CAD build for the part. Positions are in the model's coordinates, mm. Face numbers are marked on the shaded views. A direction names the side the tool comes from. Round coordinates to 2 decimals unless told otherwise and drop trailing zeros. Loops run counter-clockwise (first coordinate to the right, second up) from the corner with the lowest first, then second, coordinate; pieces in that order, holes last.
```python
from build123d import *

# Parameters (mm, degrees)
SKETCH1_R                    = 27.5
BOSS_EXTRUDE1_DEPTH          = 50
SKETCH2_R                    = 67.5
SKETCH2_R_2                  = 14
BOSS_EXTRUDE2_DEPTH          = 28
SKETCH3_R                    = 9
CUT_EXTRUDE1_DEPTH           = 12
CUT_EXTRUDE1_DRAFT           = -7.5
CUT_EXTRUDE1_PROFILE_2_DEPTH = 12
CUT_EXTRUDE1_PROFILE_2_DRAFT = -7.5
CUT_EXTRUDE1_PROFILE_3_DEPTH = 12
CUT_EXTRUDE1_PROFILE_3_DRAFT = -7.5
SKETCH4_R                    = 14
CUT_EXTRUDE2_DEPTH           = 16
CUT_EXTRUDE3_START           = -50
CUT_EXTRUDE3_DEPTH           = 50


with BuildPart() as part:
    # Sketch1 → Boss-Extrude1 (new body)
    with BuildSketch(Plane.XY):
        Circle(SKETCH1_R)
        with BuildLine():
            Line((-5, 20.8), (5, 20.8))
            Line((5, 20.8), (5, 16.770509831))
            ThreePointArc((5, 16.770509831), (0, -17.5), (-5, 16.770509831))
            Line((-5, 16.770509831), (-5, 20.8))
        make_face(mode=Mode.SUBTRACT)
    extrude(amount=BOSS_EXTRUDE1_DEPTH)

    # Sketch2 → Boss-Extrude2 (add)
    with BuildSketch(Plane(origin=(0, 0, 0), x_dir=(-1, 0, 0), z_dir=(0, 0, -1))):
        Circle(SKETCH2_R)
        with Locations((0, 45)):
            Circle(SKETCH2_R_2, mode=Mode.SUBTRACT)
        with Locations((38.97114317, -22.5)):
            Circle(SKETCH2_R_2, mode=Mode.SUBTRACT)
        with Locations((-38.97114317, -22.5)):
            Circle(SKETCH2_R_2, mode=Mode.SUBTRACT)
    extrude(amount=-BOSS_EXTRUDE2_DEPTH)


with BuildPart() as cut_extrude1_tool:
    # Sketch3 → Cut-Extrude1 (with draft: the straight prism first)
    with BuildSketch(Plane(origin=(0, 0, 0), x_dir=(-1, 0, 0), z_dir=(0, 0, -1))):
        with Locations((0, -45)):
            Circle(SKETCH3_R)
    extrude(amount=-CUT_EXTRUDE1_DEPTH)
    # Cut-Extrude1: the draft: its side faces are tilted about the plane it starts from
    cut_extrude1_sides = [cut_extrude1_tool.faces().sort_by_distance(p)[0] for p in [
        (9, -45, 6),
    ]]
    draft(cut_extrude1_sides, Plane(origin=(0, 0, 0), x_dir=(-1, 0, 0), z_dir=(0, 0, -1)), CUT_EXTRUDE1_DRAFT)


with BuildPart() as part_1:
    add(part.part)

    # Cut-Extrude1: cut by cut_extrude1_tool
    add(cut_extrude1_tool.part, mode=Mode.SUBTRACT)


with BuildPart() as cut_extrude1_profile_2_tool:
    # Sketch3 → Cut-Extrude1 profile 2 (with draft: the straight prism first)
    with BuildSketch(Plane(origin=(0, 0, 0), x_dir=(-1, 0, 0), z_dir=(0, 0, -1))):
        with Locations((-38.97114317, 22.5)):
            Circle(SKETCH3_R)
    extrude(amount=-CUT_EXTRUDE1_PROFILE_2_DEPTH)
    # Cut-Extrude1 profile 2: the draft: its side faces are tilted about the plane it starts from
    cut_extrude1_profile_2_sides = [cut_extrude1_profile_2_tool.faces().sort_by_distance(p)[0] for p in [
        (47.97114317, 22.5, 6),
    ]]
    draft(cut_extrude1_profile_2_sides, Plane(origin=(0, 0, 0), x_dir=(-1, 0, 0), z_dir=(0, 0, -1)), CUT_EXTRUDE1_PROFILE_2_DRAFT)


with BuildPart() as part_2:
    add(part_1.part)

    # Cut-Extrude1 profile 2: cut by cut_extrude1_profile_2_tool
    add(cut_extrude1_profile_2_tool.part, mode=Mode.SUBTRACT)


with BuildPart() as cut_extrude1_profile_3_tool:
    # Sketch3 → Cut-Extrude1 profile 3 (with draft: the straight prism first)
    with BuildSketch(Plane(origin=(0, 0, 0), x_dir=(-1, 0, 0), z_dir=(0, 0, -1))):
        with Locations((38.97114317, 22.5)):
            Circle(SKETCH3_R)
    extrude(amount=-CUT_EXTRUDE1_PROFILE_3_DEPTH)
    # Cut-Extrude1 profile 3: the draft: its side faces are tilted about the plane it starts from
    cut_extrude1_profile_3_sides = [cut_extrude1_profile_3_tool.faces().sort_by_distance(p)[0] for p in [
        (-29.97114317, 22.5, 6),
    ]]
    draft(cut_extrude1_profile_3_sides, Plane(origin=(0, 0, 0), x_dir=(-1, 0, 0), z_dir=(0, 0, -1)), CUT_EXTRUDE1_PROFILE_3_DRAFT)


with BuildPart() as part_3:
    add(part_2.part)

    # Cut-Extrude1 profile 3: cut by cut_extrude1_profile_3_tool
    add(cut_extrude1_profile_3_tool.part, mode=Mode.SUBTRACT)

    # Sketch4 → Cut-Extrude2 (cut)
    with BuildSketch(Plane.XY.offset(28)):
        with Locations((0, -45)):
            Circle(SKETCH4_R)
        with Locations((-38.97114317, 22.5)):
            Circle(SKETCH4_R)
        with Locations((38.97114317, 22.5)):
            Circle(SKETCH4_R)
    extrude(amount=-CUT_EXTRUDE2_DEPTH, mode=Mode.SUBTRACT)

    # Sketch7 → Cut-Extrude3 (cut)
    with BuildSketch(Plane.XY.offset(28).offset(CUT_EXTRUDE3_START)):
        with BuildLine():
            Line((-5, 16.770509831), (-5, 20.8))
            Line((-5, 20.8), (5, 20.8))
            Line((5, 20.8), (5, 16.770509831))
            ThreePointArc((5, 16.770509831), (0, -17.5), (-5, 16.770509831))
        make_face()
    extrude(amount=CUT_EXTRUDE3_DEPTH, mode=Mode.SUBTRACT)


solid = part_3.part
```
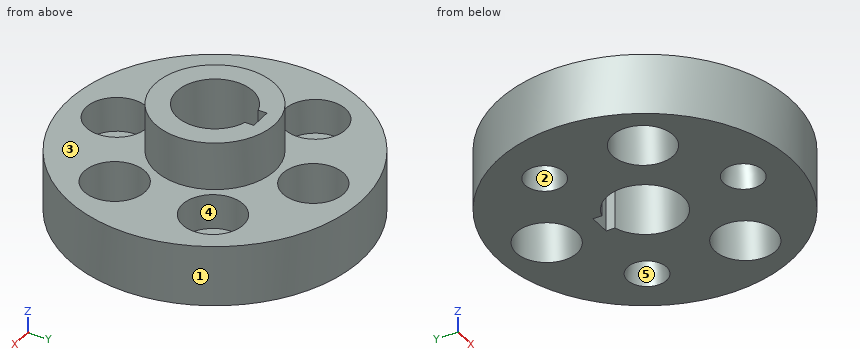
Item 1: Cut at A-A, the plane z = 19. Give the cut face in (x, y).
Answers follow:
outline: circle Ø135 at (0, 0); hole circle Ø28 at (-38.97, -22.5); hole circle Ø28 at (-38.97, 22.5); hole circle Ø28 at (0, -45); hole circle Ø28 at (0, 45); hole (-5, 16.77) arc R17.5 ccw (long way) to (5, 16.77) - (5, 20.8) - (-5, 20.8) - close; hole circle Ø28 at (38.97, -22.5); hole circle Ø28 at (38.97, 22.5)
Item 2: Cut at B-B, the plane x = 0. Give the cut face in (y, z).
Answers follow:
outline: (-67.5, 0) - (-54, 0) - (-52.42, 12) - (-59, 12) - (-59, 28) - (-67.5, 28) - close; (-37.58, 12) - (-36, 0) - (-17.5, 0) - (-17.5, 50) - (-27.5, 50) - (-27.5, 28) - (-31, 28) - (-31, 12) - close; (20.8, 0) - (31, 0) - (31, 28) - (27.5, 28) - (27.5, 50) - (20.8, 50) - close; (59, 0) - (67.5, 0) - (67.5, 28) - (59, 28) - close
Item 3: Two-plate mould, pull along X, no slides. Class the marked faces 1, 2 and 3: released by +X, released by -X, zero draft, split by the parting line, or undercut.
Answers follow:
face 1: split by the parting line
face 2: undercut
face 3: zero draft
Item 4: Probe line 1 (X direction, y = 26.5, z = 3); line 2 (Y direction, x = 38, z = 10); line 3 (X direction, y = 22, z = 19). List the from-to ranges inside material, lowest first.
Answers follow:
line 1: x = -62.08 to -46.59, -31.35 to 31.35, 46.59 to 62.08
line 2: y = -55.79 to -36.47, -8.53 to 14.88, 30.12 to 55.79
line 3: x = -63.81 to -52.96, -24.98 to 24.98, 52.96 to 63.81
Item 5: 3-axis set-ups, long thin cutter, end or side, ignore diameter. For the marked faces 4 and 5: which of +Z, -Z, +X, -X, +Y, -Y reach the whole face in a straight line?
Answers follow:
face 4: +Z
face 5: -Z
Item 6: Cut at C-C, the plane y = -45. Give the cut face in (x, z).
Answers follow:
outline: (-50.31, 0) - (-9, 0) - (-7.42, 12) - (-14, 12) - (-14, 28) - (-50.31, 28) - close; (7.42, 12) - (9, 0) - (50.31, 0) - (50.31, 28) - (14, 28) - (14, 12) - close
Item 7: Cut at D-D, the plane z = 40. Give the cut face in (x, y).
Answers follow:
outline: circle Ø55 at (0, 0); hole (-5, 16.77) arc R17.5 ccw (long way) to (5, 16.77) - (5, 20.8) - (-5, 20.8) - close
Item 8: Flat gauge pins, fed straight in: P1, Ø4, axis at x = -30, z = 43.5, coming from the -Y side; P2, Ø1.5, axis at y = -16, z = 40.5, coming from the +X side; P3, Ø10, axis at x = 25, y = 1, coming from the -Z side; P4, Ø11, axis at x = 2, z = 14.5, coming from the -Y side. Where does each tip first touch, or does it go through?
Answers follow:
P1: passes through
P2: stops at x = 22.88
P3: stops at z = 0
P4: stops at y = -67.5
